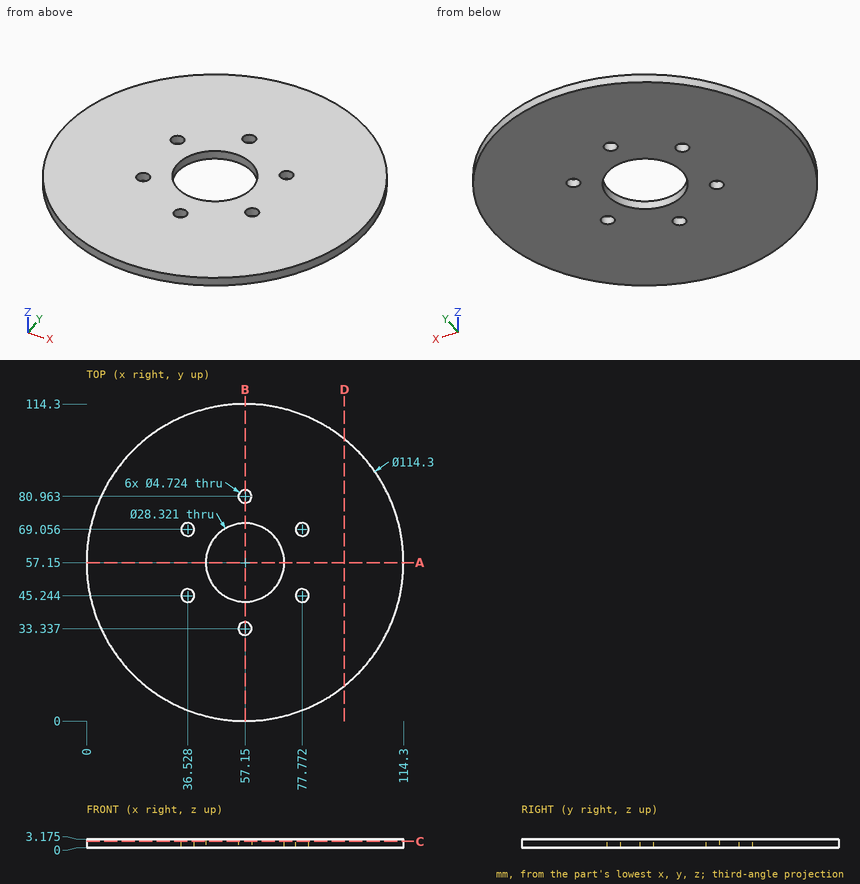
Source: three-view drawing plus pictorial views. Frame: mm from the lowest corner of the part. Round coordinates to 2 decimals unless told otherwise and drop trailing zeros. Loops run counter-clockwise (first coordinate to the right, second up) from the corner with the lowest first, then second, coordinate; pieces in that order, holes last. Notation, with made-up numbers: M 58.5,-5.75 L 117.5,-5.75 A16 cw 117.5,-0.75 Z; hole C -34,43 d4. An arc over 180 degrees is marked long. Answer as CSV lines item,"result".
Q1. Cut plane A-A (y = 57.15). Return the cut outline in (x, z) (1 decimal), plus the area to 3 significant figures.
Verdict:
outline,"M 0,0 L 43,0 L 43,3.2 L 0,3.2 Z; M 71.3,0 L 114.3,0 L 114.3,3.2 L 71.3,3.2 Z"
area,"273 mm^2"
Q2. Cut plane B-B (x = 57.15). Return the cut outline in (y, z) (1 decimal).
Verdict:
outline,"M 0,0 L 31,0 L 31,3.2 L 0,3.2 Z; M 35.7,0 L 43,0 L 43,3.2 L 35.7,3.2 Z; M 71.3,0 L 78.6,0 L 78.6,3.2 L 71.3,3.2 Z; M 83.3,0 L 114.3,0 L 114.3,3.2 L 83.3,3.2 Z"
Q3. Line query: line 1 along Y through (x, z) = (57.15, 2.2) (1 decimal); line 2 along X through (y, z) = (69, 2.1) (1 decimal); line 3 along X through (y, z) = (34.5, 1.8) (1 decimal). Output: solid intervals per line, ascending.
Verdict:
line 1,"y = 0 to 31, 35.7 to 43, 71.3 to 78.6, 83.3 to 114.3"
line 2,"x = 1.2 to 34.2, 38.9 to 49.4, 64.9 to 75.4, 80.1 to 113.1"
line 3,"x = 4.7 to 55.1, 59.2 to 109.6"
Q4. Cut plane D-D (x = 93). Return the cut outline in (y, z) (1 decimal).
Verdict:
outline,"M 12.6,0 L 101.7,0 L 101.7,3.2 L 12.6,3.2 Z"
Q5. Contact query for flat-ended pins moving along their axis: pin 1 (3 mm diameter, centred on x = 57.15, y = 33.34, fed in from -Z); pin 2 (1 mm diameter, centred on y = 17, z = 2.5, fed in from -X). Output: stop coordinate, or through.
Verdict:
pin 1,"passes through"
pin 2,"stops at x = 15.99"
Q6. Cut plane C-C (z = 2.3). Count the separate pieces of the cut face and the enclosed holes in it, plus the area to 3 significant figures.
Verdict:
separate pieces,"1"
enclosed holes,"7"
area,"9,530 mm^2"
